Part model, mm, in its own coordinate system. A direction names the side the tool comes from. Coordinates: 2 decimals unless noted, no trailing zeros. Write each loop counter-clockwise with the first axis right and the second up, starting at its lowest first coordinate (ties: lowest second). Pieces come first, ordered by that corner, then holes. Notation, with made-up numbers: M 80,43.25 L 108,43.25 A18 ccw 108,52.25 Z; hole C -3.5,71.25 d8. An arc over 180 degrees is marked long. Use a Markdown table: item, result. Add a question column.
Q1. Slice it at A-A on x = 218.5. Write the cut outline in (y, z), then the cut area to 3 significant figures.
Q2. Slice it at B-B on z = -5.75. Write the cut outline in (x, y).
Q3. Mould opens along Y. For faces 1 (the flat face through (446, -12.7, 0)), 2 (the flat face through (0, -0.2, 11.5)), 3 (the flat face through (446, 0, 11.049)), 4 (the flat face through (446, 12.7, 0)) say: released by +Y, released by -Y, zero draft, split by the parting line, or undercut.
Q4. Pin check, flat tip, straight feed: pin 1 Ø6 at (y, z) = (9.5, -1.5) entering from +X. Stop position of the tip, or through.
Q5. Tool access for faces 5 (the flat face through (446, 11.049, 0)), 6 (the flat face through (446, 0, 12.7)): list every direction of +Z, -Z, +X, -X, +Y, -Y with a clear straight run to the whole face (end or side of a thin tool).
Q6. Wall check: L1, parallel to Y at x = 705, z = -3. Give the ranges that are in metal, low to high. Write a range as from..to.
from build123d import *

# Parameters (mm, degrees)
SKETCH13_W                                     = 25.4
SKETCH13_H                                     = 25.4
SKETCH13_W_2                                   = 22.098
SKETCH13_H_2                                   = 22.098
AL_TUBE_SQUARE_AL_TUBE_1_SQR_X_0_065_WAL_DEPTH = 905.4


with BuildPart() as part:
    # Sketch13 → Al tube square AL TUBE 1 SQR X 0.065 WALL(1) (new body)
    with BuildSketch(Plane.YZ):
        Rectangle(SKETCH13_W, SKETCH13_H)
        Rectangle(SKETCH13_W_2, SKETCH13_H_2, mode=Mode.SUBTRACT)
    extrude(amount=AL_TUBE_SQUARE_AL_TUBE_1_SQR_X_0_065_WAL_DEPTH)


solid = part.part
Recorded:
| question | item | result |
|---|---|---|
| 1 | outline | M -12.7,-12.7 L 12.7,-12.7 L 12.7,12.7 L -12.7,12.7 Z; hole M -11.05,-11.05 L 11.05,-11.05 L 11.05,11.05 L -11.05,11.05 Z |
| 1 | area | 157 mm² |
| 2 | outline | M 0,-12.7 L 905.4,-12.7 L 905.4,-11.05 L 0,-11.05 Z; M 0,11.05 L 905.4,11.05 L 905.4,12.7 L 0,12.7 Z |
| 3 | face 1 | released by -Y |
| 3 | face 2 | zero draft |
| 3 | face 3 | undercut |
| 3 | face 4 | released by +Y |
| 4 | pin 1 | x = 905.4 |
| 5 | face 5 | +X, -X |
| 5 | face 6 | +Z, +X, -X, +Y, -Y |
| 6 | L1 | -12.7..-11.05, 11.05..12.7 |
